Autodesk Inventor part; units mm, degrees
ref_plane "YZ Plane" through (0, 0, 0) normal (1, 0, 0) x (0, 1, 0)
ref_plane "XZ Plane" through (0, 0, 0) normal (0, 1, 0) x (-1, 0, 0)
ref_plane "XY Plane" through (0, 0, 0) normal (0, 0, 1) x (1, 0, 0)
sketch "Sketch1" plane through (0, 0, 0) normal (0, 0, 1) x (1, 0, 0)
  line L0 (-28.448, 28.448) -> (28.448, 28.448)
  line L1 (28.448, 28.448) -> (28.448, -28.448)
  line L2 (28.448, -28.448) -> (-28.448, -28.448)
  line L3 (-28.448, -28.448) -> (-28.448, 28.448)
  point P0 (0, 0)
  point P1 (-28.448, 0)
  point P2 (0, 28.448)
  dimension "d0" = 56.896
extrude "Extrusion1" add sketch "Sketch1" along normal blind 12.7
sketch "Sketch2" plane through (0, 0, 12.7) normal (0, 0, 1) x (1, 0, 0)
  circle A0 centre (0, 0) radius 21.844
  dimension "d4" = 43.688
extrude "Extrusion2" add sketch "Sketch2" along normal blind 24.638
sketch "Sketch3" plane through (0, 0, 37.338) normal (0, 0, 1) x (1, 0, 0)
  circle A0 centre (0, 0) radius 21.844
  circle A1 centre (0, 0) radius 6
  dimension "d8" = 12
extrude "Extrusion3" add sketch "Sketch3" along normal blind 30.64 contours A1
thread "Thread1"
sketch "Sketch4" plane through (0, 0, 0) normal (0, 0, -1) x (-1, 0, 0)
  circle A0 centre (0, 0) radius 23.425
  dimension "d14" = 46.85
extrude "Extrusion4" add sketch "Sketch4" along normal blind 11.25
fillet "Fillet1" radius 3.175 4 edges at (28.448, 28.448, 6.35) (-28.448, 28.448, 6.35) (28.448, -28.448, 6.35) (-28.448, -28.448, 6.35)
sketch "Sketch5" plane through (0, 0, -11.25) normal (0, 0, -1) x (-1, 0, 0)
  circle A0 centre (0, 0) radius 23.425
  circle A1 centre (0, 0) radius 17.5
  dimension "d21" = 35
extrude "Extrusion5" add sketch "Sketch5" along normal blind 48.05 contours A1
sketch "Sketch6" plane through (0, 0, 12.7) normal (0, 0, 1) x (1, 0, 0)
  line L0 (28.448, -25.273) -> (28.448, 25.273)
  line L1 (25.273, 28.448) -> (-25.273, 28.448)
  line L2 (-28.448, 25.273) -> (-28.448, -25.273)
  line L3 (21.2598, 21.2598) -> (21.2598, -21.2598)
  line L4 (-21.2598, 21.2598) -> (21.2598, 21.2598)
  point P0 (-21.2598, -21.2598)
  point P1 (0, 21.2598)
  point P2 (0, 28.448)
  point P3 (21.2598, 0)
  point P4 (28.448, 0)
  dimension "d25" = 42.5196
  dimension "d27" = 42.5196
hole "Hole1" at (-21.2598, 21.2598, 12.7) at (21.2598, 21.2598, 12.7) at (21.2598, -21.2598, 12.7) at (-21.2598, -21.2598, 12.7) direction (0, 0, -1) diameter 5.5 end through all
sketch "Sketch7" plane through (0, 0, 37.338) normal (0, 0, 1) x (1, 0, 0)
  circle A0 centre (0, 0) radius 6
  circle A1 centre (0, 0) radius 21.844
  circle A2 centre (0, 0) radius 12.7
  dimension "d35" = 25.4
extrude "Extrusion6" add sketch "Sketch7" along normal blind 2.286 contours A2
properties part number "Pg_15"
Geometry: final body of the model. Coordinates: model frame, mm. A direction names the side the tool comes from. Round coordinates to 2 decimals unless told otherwise and drop trailing zeros. Order: outer loops, then holes, each group sorted by start corner. A loop starts at its lowest first (then second) coordinate and runs counter-clockwise, first axis right, second up.
Q1. Section C-C, the plane z = -42.5. Output: boundary loops of the cut face in (x, y), and give its area (3 significant figures).
Result sheet:
outline: circle Ø35 at (0, 0)
area: 962 mm2
Q2. Pin query (flat end, axial travel): pin 1 (1 mm diameter, centred on y = -7, z = 23.5, fed in from +X); pin 2 (7 mm diameter, centred on x = 21.26, y = -21.26, fed in from +Z); pin 3 (6 mm diameter, centred on y = -21.5, z = 38.5, fed in from +X). Return the tip coordinate at first contact, or that it passes through.
Result sheet:
pin 1: stops at x = 20.85
pin 2: stops at z = 12.7
pin 3: stops at x = 11.23
Q3. Material intervals for probe 1 along Z at (x, y) = (-21, 10); probe 2 along Z at (x, y) = (-13.5, 25.5); probe 3 along X at (y, z) = (-3.5, -31.5), sorted ascending.
Result sheet:
probe 1: z = -11.25 to 12.7
probe 2: z = 0 to 12.7
probe 3: x = -17.15 to 17.15
Q4. Section D-D, the plane x = -8. Output: boundary loops of the cut face in (y, z).
Result sheet:
outline: (-28.45, 0) - (-22.02, 0) - (-22.02, -11.25) - (-15.56, -11.25) - (-15.56, -59.3) - (15.56, -59.3) - (15.56, -11.25) - (22.02, -11.25) - (22.02, 0) - (28.45, 0) - (28.45, 12.7) - (20.33, 12.7) - (20.33, 37.34) - (9.86, 37.34) - (9.86, 39.62) - (-9.86, 39.62) - (-9.86, 37.34) - (-20.33, 37.34) - (-20.33, 12.7) - (-28.45, 12.7) - close
Q5. Section A-A, the plane x = 0. Output: boundary loops of the cut face in (y, z) (3 decimals), and give its area (3 significant figures).
Result sheet:
outline: (-28.448, 0) - (-23.425, 0) - (-23.425, -11.25) - (-17.5, -11.25) - (-17.5, -59.3) - (17.5, -59.3) - (17.5, -11.25) - (23.425, -11.25) - (23.425, 0) - (28.448, 0) - (28.448, 12.7) - (21.844, 12.7) - (21.844, 37.338) - (12.7, 37.338) - (12.7, 39.624) - (6, 39.624) - (6, 67.978) - (-6, 67.978) - (-6, 39.624) - (-12.7, 39.624) - (-12.7, 37.338) - (-21.844, 37.338) - (-21.844, 12.7) - (-28.448, 12.7) - close
area: 4,410 mm2
Q6. Access query for faces 5 (the face through (13.887, 10.648, -34.939)), 6 (the face through (23.944, -20.664, 6.261)), 7 (the face through (9.4, -9.4, 37.338)). Directions: +Z, -Z, +X, -X, +Y, -Y. A direction counts if a zero-diameter tool reaches every point of the face in a straight line with its end or side. Return the directions, or none.
Result sheet:
face 5: -Z
face 6: +Z, -Z
face 7: +Z
Q7. Mould query, pull axis Y, two halves, no side actions, for faces 1 (the face through (28.448, 0, 6)), 2 (the face through (-23.986, -20.902, 6.261)), 3 (the face through (18.59, 14.25, -5.55)), 4 (the face through (23.944, 21.856, 6.261)). Classes: released by +Y, released by -Y, zero draft, split by the parting line, or undercut.
Result sheet:
face 1: zero draft
face 2: undercut
face 3: split by the parting line
face 4: undercut
